Job drawing, mm, ordinate dimensions from the low corner. One solid piece. Round coordinates to 2 decimals unless told otherwise and drop trailing zeros. Loops run counter-clockwise (first coordinate to the right, second up) from the corner with the lowest first, then second, coordinate; pieces in that order, holes last.
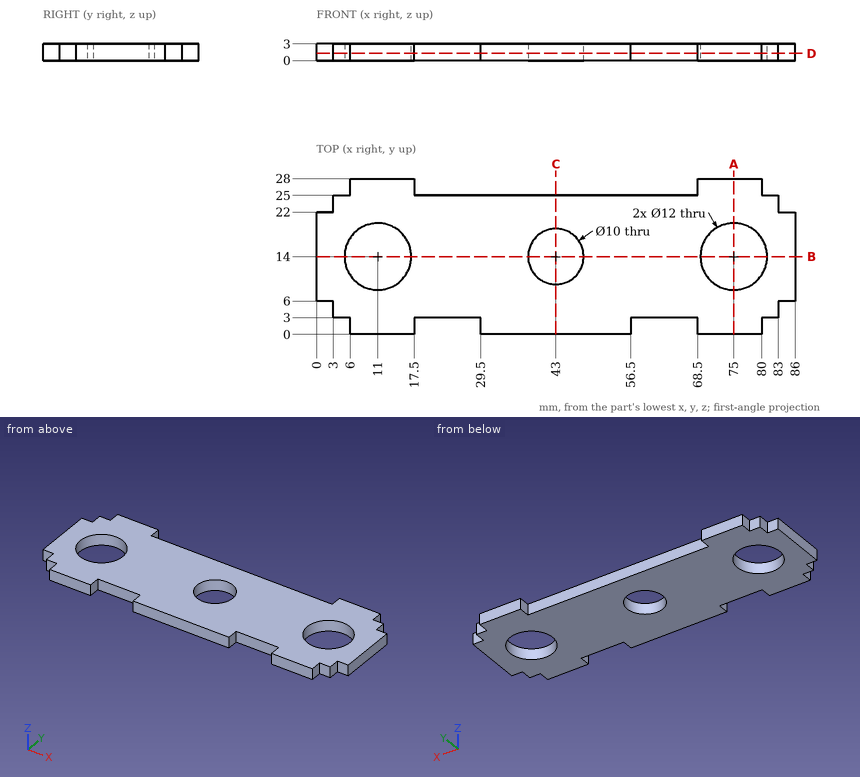
Item 1: Probe line 1 (X direction, y = 14.25, z = 2.3); line 2 (Y direction, x = 75, z = 1.9); line 3 (X direction, y = 1.75, z = 1.9). List the from-to ranges inside material, lowest first.
Answers follow:
line 1: x = 0 to 5.01, 16.99 to 38.01, 47.99 to 69.01, 80.99 to 86
line 2: y = 0 to 8, 20 to 28
line 3: x = 6 to 17.5, 29.5 to 56.5, 68.5 to 80
Item 2: Flat gauge pins, fed straight in: P1, Ø0.9, axis at y = 26.5, z = 1, coming from the -X side; P2, Ø1.5, axis at y = 26, z = 1.5, coming from the +X side; P3, Ø0.9, axis at x = 85, z = 1.5, coming from the -Y side. Where does each tip first touch, or does it go through?
Answers follow:
P1: stops at x = 6
P2: stops at x = 80
P3: stops at y = 6
Item 3: Cut at C-C, the plane x = 43. Give the cut face in (y, z), plus the area to 3 significant figures.
Answers follow:
outline: (0, 0) - (9, 0) - (9, 3) - (0, 3) - close; (19, 0) - (25, 0) - (25, 3) - (19, 3) - close
area: 45.0 mm2
Item 4: Cut at D-D, the plane z = 1.3. State how many separate pieces and enclosed holes the cut face has, plus the area to 3 significant figures.
Answers follow:
separate pieces: 1
enclosed holes: 3
area: 1,770 mm2
Item 5: Cut at A-A, the plane x = 75. Give the cut face in (y, z).
Answers follow:
outline: (0, 0) - (8, 0) - (8, 3) - (0, 3) - close; (20, 0) - (28, 0) - (28, 3) - (20, 3) - close
Item 6: Cut at B-B, the plane y = 14. Give the cut face in (x, z), plus the area to 3 significant figures.
Answers follow:
outline: (0, 0) - (5, 0) - (5, 3) - (0, 3) - close; (17, 0) - (38, 0) - (38, 3) - (17, 3) - close; (48, 0) - (69, 0) - (69, 3) - (48, 3) - close; (81, 0) - (86, 0) - (86, 3) - (81, 3) - close
area: 156 mm2
